from build123d import *

# Parameters (mm, degrees)
SKETCH2_R           = 1.5
BOSS_EXTRUDE1_DEPTH = 5
SKETCH3_W           = 147
SKETCH3_H           = 3
BOSS_EXTRUDE2_DEPTH = 3
FILLET1_R           = 10
FILLET2_R           = 10
SKETCH4_W           = 194.268756053
SKETCH4_H           = 72.725923545
SKETCH4_W_2         = 127
SKETCH4_H_2         = 5
CUT_EXTRUDE1_DEPTH  = 10


with BuildPart() as part:
    # Sketch2 → Boss-Extrude1 (new body)
    with BuildSketch(Plane(origin=(0, 0, 0), x_dir=(1, 0, 0), z_dir=(0, 1, 0))):
        Polygon((79.832898172, 11.229765013), (51.332898172, 11.229765013), (9.722898172, 11.229765013), (-67.167101828, 11.229765013), (-67.167101828, 37.229765013), (79.832898172, 37.229765013), align=None)
        with Locations(Location((9.722898172, 17.579765013, 0), (0, 0, 270))):
            Circle(SKETCH2_R, mode=Mode.SUBTRACT)
        with Locations(Location((51.332898172, 17.579765013, 0), (0, 0, 270))):
            Circle(SKETCH2_R, mode=Mode.SUBTRACT)
        with Locations(Location((-50.267101828, 17.579765013, 0), (0, 0, 270))):
            Circle(SKETCH2_R, mode=Mode.SUBTRACT)
    extrude(amount=BOSS_EXTRUDE1_DEPTH)

    # Sketch3 → Boss-Extrude2 (add)
    with BuildSketch(Plane(origin=(0, 5, 0), x_dir=(1, 0, 0), z_dir=(0, 1, 0))):
        with Locations((6.332898172, 25.729765013)):
            Rectangle(SKETCH3_W, SKETCH3_H)
    extrude(amount=BOSS_EXTRUDE2_DEPTH)

    # Fillet1
    fillet1_edges = [part.edges().sort_by_distance(p)[0] for p in [
        (-67.167101828, 2.5, -37.229765013),
        (-67.167101828, 2.5, -11.229765013),
    ]]
    fillet(fillet1_edges, radius=FILLET1_R)

    # Fillet2
    fillet2_edges = [part.edges().sort_by_distance(p)[0] for p in [
        (79.832898172, 2.5, -37.229765013),
        (79.832898172, 2.5, -11.229765013),
    ]]
    fillet(fillet2_edges, radius=FILLET2_R)

    # Sketch4 → Cut-Extrude1 (cut)
    # profile 1 of 2: a face of its own
    with BuildSketch(Plane(origin=(0, 0, -37.229765013), x_dir=(-1, 0, 0), z_dir=(0, 0, -1))):
        with Locations((1.63687335, -5.593113251)):
            Rectangle(SKETCH4_W, SKETCH4_H)
        with Locations((-6.332898172, 2.5)):
            Rectangle(SKETCH4_W_2, SKETCH4_H_2, mode=Mode.SUBTRACT)
    # profile 2 of 2: a face of its own
    with BuildSketch(Plane(origin=(0, 0, -37.229765013), x_dir=(-1, 0, 0), z_dir=(0, 0, -1))):
        with Locations((-6.332898172, 2.5)):
            Rectangle(SKETCH4_W_2, SKETCH4_H_2)
    extrude(amount=-CUT_EXTRUDE1_DEPTH, mode=Mode.SUBTRACT)


solid = part.part
Model file for the job. Use its own axes, mm. A direction names the side the tool comes from. Round coordinates to 2 decimals unless told otherwise and drop trailing zeros. Order: outer loops, then holes, each group sorted by start corner. A loop starts at its lowest first (then second) coordinate and runs counter-clockwise, first axis right, second up.
(1) Pull direction X, two halves, no side cores. Call faces 1 (the face through (-49.82, 2.46, -16.15)), 2 (the face through (-67.167, 3, -24)), 3 (the face through (7, 4, -27.23)), 4 (the face through (52.82, 2.46, -17.78)): released by +X, released by -X, zero draft, split by the parting line, or undercut.
(2) 3-axis set-ups, long thin cutter, end or side, ignore diameter. For faces 5 (the face through (-64.16, 2.54, -14.08)), 6 (the face through (5, 6, -24.23)): which of +Z, -Z, +X, -X, +Y, -Y reach the whole face in a straight line?
(3) Band-saw the part on B-B (y = 3.25). List the corners of the cut face in (x, z), then the cut area to 3 significant figures.
(4) Band-saw the part on A-A (x = -2). List the corners of the cut face in (y, z), then the cut area to 3 significant figures.
(5) Drill centre lines: line 1 (X direction, y = 4, z = -18.75); line 2 (Y direction, x = -18, z = -17.5); line 3 (Z direction, x = 8.5, y = 4). Where is each one in solid material? Low to high.
(6) Pin check, flat tips, straight feed: pin 1 (4 mm diameter, centred on y = 6.5, z = -20, fed in from -X); pin 2 (2.5 mm diameter, centred on x = 2.5, y = 7, fed in from +Z); pin 3 (4 mm diameter, centred on x = -24, z = -19.5, fed in from +Y); pin 4 (3 mm diameter, centred on y = 5.5, z = -14.5, fed in from -X). Stop position of each tip, or through.
(7) Band-saw the part on C-C (z = -14). List the corners of the cut face in (x, y), then the cut area to 3 significant figures.
Verdict:
1. face 1: undercut
1. face 2: released by -X
1. face 3: zero draft
1. face 4: undercut
2. face 5: +Z, -X, +Y, -Y
2. face 6: +Z, +X, -X, +Y
3. outline: (-67.17, -27.23) - (79.83, -27.23) - (79.83, -21.23) arc R10 ccw to (69.83, -11.23) - (-57.17, -11.23) arc R10 ccw to (-67.17, -21.23) - close; hole circle Ø3 at (-50.27, -17.58); hole circle Ø3 at (9.72, -17.58); hole circle Ø3 at (51.33, -17.58)
3. area: 2,290 mm2
4. outline: (0, -27.23) - (8, -27.23) - (8, -24.23) - (5, -24.23) - (5, -11.23) - (0, -11.23) - close
4. area: 89.0 mm2
5. line 1: x = -66.85 to -51.21, -49.33 to 8.78, 10.66 to 50.39, 52.27 to 79.52
5. line 2: y = 0 to 5
5. line 3: z = -27.23 to -18.45, -16.71 to -11.23
6. pin 1: stops at x = -67.17
6. pin 2: stops at z = -24.23
6. pin 3: stops at y = 5
6. pin 4: stops at x = -65.64
7. outline: (-64.08, 0) - (76.74, 0) - (76.74, 5) - (-64.08, 5) - close
7. area: 704 mm2
